Here's how the part is built. I have some questions about the finished solid (model axes, mm). A direction names the side the tool comes from. Coordinates: 2 decimals unless noted, no trailing zeros. Write each loop counter-clockwise with the first axis right and the second up, starting at its lowest first coordinate (ties: lowest second). Pieces come first, ordered by that corner, then holes.
```python
from build123d import *

# Parameters (mm, degrees)
SKETCH_1_W                         = 320
SKETCH_1_H                         = 22
SM_BASE_FLANGE_1_DEPTH             = 2
SM_EDGE_FLANGE_1_STRIP_W           = 10
SM_EDGE_FLANGE_1_STRIP_H           = 2
SM_EDGE_FLANGE_1_STRIP_CUT_DEPTH   = 320
SM_EDGE_FLANGE_1_STRIP_2_W         = 10
SM_EDGE_FLANGE_1_STRIP_2_H         = 2
SM_EDGE_FLANGE_1_STRIP_CUT_2_DEPTH = 320
SM_EDGE_FLANGE_1_DEPTH             = 320
SM_EDGE_FLANGE_1_BEND_DEPTH        = 320
SM_EDGE_FLANGE_2_STRIP_W           = 10
SM_EDGE_FLANGE_2_STRIP_H           = 2
SM_EDGE_FLANGE_2_STRIP_CUT_DEPTH   = 16
SM_EDGE_FLANGE_2_STRIP_2_W         = 10
SM_EDGE_FLANGE_2_STRIP_2_H         = 2
SM_EDGE_FLANGE_2_STRIP_CUT_2_DEPTH = 16
SM_EDGE_FLANGE_2_DEPTH             = 16
SM_EDGE_FLANGE_2_BEND_DEPTH        = 16
SKETCH_18_W                        = 9
SKETCH_18_H                        = 9
CUT_EXTRUDE_1_DEPTH                = 10
PATTERN_LINEAR_1_COUNT             = 20
PATTERN_LINEAR_1_PITCH             = 20


# Sheet-metal steps are written as plain solids
with BuildPart() as part:
    # Sketch 1 → 基体-法兰1 (new body)
    with BuildSketch(Plane.XY):
        Rectangle(SKETCH_1_W, SKETCH_1_H)
    extrude(amount=-SM_BASE_FLANGE_1_DEPTH)

    # 边线-法兰1 strip (across the edge) → 边线-法兰1 strip cut (cut)
    with BuildSketch(Plane(origin=(160, -11, -2), x_dir=(0, 1, 0), z_dir=(-1, 0, 0))):
        with Locations((-2, -1)):
            Rectangle(SM_EDGE_FLANGE_1_STRIP_W, SM_EDGE_FLANGE_1_STRIP_H)
    extrude(amount=SM_EDGE_FLANGE_1_STRIP_CUT_DEPTH, mode=Mode.SUBTRACT)

    # 边线-法兰1 strip 2 (across the edge) → 边线-法兰1 strip cut 2 (cut)
    with BuildSketch(Plane(origin=(-160, 11, -2), x_dir=(0, -1, 0), z_dir=(1, 0, 0))):
        with Locations((-2, -1)):
            Rectangle(SM_EDGE_FLANGE_1_STRIP_2_W, SM_EDGE_FLANGE_1_STRIP_2_H)
    extrude(amount=SM_EDGE_FLANGE_1_STRIP_CUT_2_DEPTH, mode=Mode.SUBTRACT)

    # 边线-法兰1 section (across the edge) → 边线-法兰1 (add)
    with BuildSketch(Plane(origin=(160, -11, -2), x_dir=(0, 1, 0), z_dir=(-1, 0, 0))):
        with BuildLine():
            Line((0, 1), (0, 8))
            Line((0, 8), (2, 8))
            Line((2, 8), (2, 1))
            ThreePointArc((2, 1), (2.292893219, 0.292893219), (3, 0))
            Line((3, 0), (3, -2))
            ThreePointArc((3, -2), (0.878679656, -1.121320344), (0, 1))
        make_face()
    extrude(amount=SM_EDGE_FLANGE_1_DEPTH)

    # 边线-法兰1 section 2 (across the edge) → 边线-法兰1 bend (add)
    with BuildSketch(Plane(origin=(-160, 11, -2), x_dir=(0, -1, 0), z_dir=(1, 0, 0))):
        with BuildLine():
            Line((0, 1), (0, 8))
            Line((0, 8), (2, 8))
            Line((2, 8), (2, 1))
            ThreePointArc((2, 1), (2.292893219, 0.292893219), (3, 0))
            Line((3, 0), (3, -2))
            ThreePointArc((3, -2), (0.878679656, -1.121320344), (0, 1))
        make_face()
    extrude(amount=SM_EDGE_FLANGE_1_BEND_DEPTH)

    # 边线-法兰2 strip (across the edge) → 边线-法兰2 strip cut (cut)
    with BuildSketch(Plane(origin=(-160, -8, -2), x_dir=(1, 0, 0), z_dir=(0, 1, 0))):
        with Locations((-2, -1)):
            Rectangle(SM_EDGE_FLANGE_2_STRIP_W, SM_EDGE_FLANGE_2_STRIP_H)
    extrude(amount=SM_EDGE_FLANGE_2_STRIP_CUT_DEPTH, mode=Mode.SUBTRACT)

    # 边线-法兰2 strip 2 (across the edge) → 边线-法兰2 strip cut 2 (cut)
    with BuildSketch(Plane(origin=(160, 8, -2), x_dir=(-1, 0, 0), z_dir=(0, -1, 0))):
        with Locations((-2, -1)):
            Rectangle(SM_EDGE_FLANGE_2_STRIP_2_W, SM_EDGE_FLANGE_2_STRIP_2_H)
    extrude(amount=SM_EDGE_FLANGE_2_STRIP_CUT_2_DEPTH, mode=Mode.SUBTRACT)

    # 边线-法兰2 section (across the edge) → 边线-法兰2 (add)
    with BuildSketch(Plane(origin=(-160, -8, -2), x_dir=(1, 0, 0), z_dir=(0, 1, 0))):
        with BuildLine():
            Line((0, 1), (0, 8))
            Line((0, 8), (2, 8))
            Line((2, 8), (2, 1))
            ThreePointArc((2, 1), (2.292893219, 0.292893219), (3, 0))
            Line((3, 0), (3, -2))
            ThreePointArc((3, -2), (0.878679656, -1.121320344), (0, 1))
        make_face()
    extrude(amount=SM_EDGE_FLANGE_2_DEPTH)

    # 边线-法兰2 section 2 (across the edge) → 边线-法兰2 bend (add)
    with BuildSketch(Plane(origin=(160, 8, -2), x_dir=(-1, 0, 0), z_dir=(0, -1, 0))):
        with BuildLine():
            Line((0, 1), (0, 8))
            Line((0, 8), (2, 8))
            Line((2, 8), (2, 1))
            ThreePointArc((2, 1), (2.292893219, 0.292893219), (3, 0))
            Line((3, 0), (3, -2))
            ThreePointArc((3, -2), (0.878679656, -1.121320344), (0, 1))
        make_face()
    extrude(amount=SM_EDGE_FLANGE_2_BEND_DEPTH)

    # 草图18 → 切除-拉伸1 (cut)
    with BuildSketch(Plane.XY):
        with Locations((-150, 1)):
            Rectangle(SKETCH_18_W, SKETCH_18_H)
    cut_extrude_1 = extrude(amount=-CUT_EXTRUDE_1_DEPTH, mode=Mode.SUBTRACT)

    # 阵列(线性)1: 切除-拉伸1 ×20
    with Locations(*[(i * PATTERN_LINEAR_1_PITCH, 0, 0) for i in range(1, PATTERN_LINEAR_1_COUNT)]):
        add(cut_extrude_1, mode=Mode.SUBTRACT)


solid = part.part
```
1) I need wall thicknesses on probe 1 along X at (y, z) = (2.75, -8.25); probe 2 along Y at (x, z) = (32, -7.75); probe 3 along Z at (x, y) = (-140.5, -4). Which ranges of each line are inside material? Lowest first, please.
Values follow:
probe 1: x = -160 to -158, 158 to 160
probe 2: y = -11 to -9, 9 to 11
probe 3: z = -2 to 0
2) We'd pull the mould along X, two halves only. Please class faces 4 (the face through (-158, 0, -7)), 5 (the face through (-2, 0, -2)), 6 (the face through (160, 0, -6)), 7 (the face through (2, -9, -7)): pulls with the +X half, pulls with the -X half, needs draft (parallel to the pull), parting line crosses it, or undercut.
Values follow:
face 4: undercut
face 5: undercut
face 6: pulls with the +X half
face 7: needs draft
3) Imagine slicing it at B-B on y = 0. Count the separate pieces of the cut face and the enclosed holes in it, then the cut area to 3 significant figures.
Values follow:
separate pieces: 17
enclosed holes: 0
area: 381 mm2
4) Imagine slicing it at A-A on z = -5. Please give me the cut outline in (x, y).
Values follow:
outline: (-160, -11) - (160, -11) - (160, -9) - (-160, -9) - close; (-160, -8) - (-158, -8) - (-158, 8) - (-160, 8) - close; (-160, 9) - (160, 9) - (160, 11) - (-160, 11) - close; (158, -8) - (160, -8) - (160, 8) - (158, 8) - close
5) On a 3-axis mill with a long thin cutter (end or side, diameter ignored), from which of +Z, -Z, +X, -X, +Y, -Y can I reach the whole of each face in a straight line? I mean faces 1 (the face through (-2, 9, -7)), 2 (the face through (158, 0, -7)), 3 (the face through (-2, 11, -6)). Say none if no direction works.
Values follow:
face 1: -Z, +X, -X
face 2: -Z
face 3: +Z, -Z, +X, -X, +Y
6) Will these pins go through, and if not, where does the flat tip stop? pin 1 (1 mm diameter, centred on y = 1, z = -1, fed in from -X); pin 2 (1.6 mm diameter, centred on x = -28, z = -0.5, fed in from -Y); pin 3 (1.6 mm diameter, centred on y = -0.5, z = -0.5, fed in from +X).
Values follow:
pin 1: stops at x = -159.6
pin 2: stops at y = -10.47
pin 3: stops at x = 159.47
